Can you work these out from the drawing? Everything is in mm from the part's minimum corner. Coordinates: 2 decimals unless noted, no trailing zeros. Loops run counter-clockwise (first coordinate to the right, second up) from the corner with the lowest first, then second, coordinate; pieces in that order, holes last.
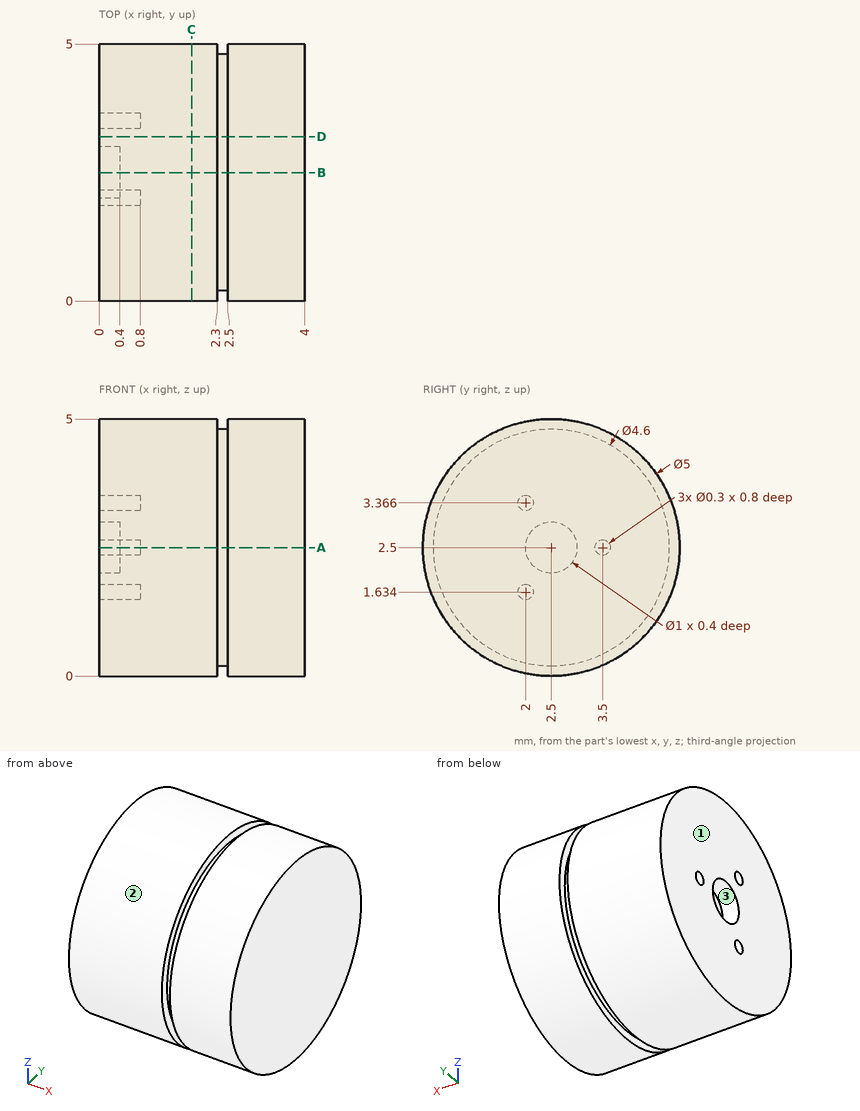
(1) We'd pull the mould along Z, two halves only. Please class the marked faces 1, 2 and 3: +Z half, -Z half, draft (parallel to the pull), parting line (faces both ways), or undercut.
Answers:
face 1: draft
face 2: parting line
face 3: undercut
(2) I need wall thicknesses on probe 1 along Y at (x, z) = (0.1, 2.5); probe 2 along Z at (x, y) = (0.3, 2.25); probe 3 along Z at (x, y) = (3.75, 2.6). Which ranges of each line are inside material? Lowest first, please.
Answers:
probe 1: y = 0 to 2, 3 to 3.35, 3.65 to 5
probe 2: z = 0.01 to 2.07, 2.93 to 4.99
probe 3: z = 0 to 5
(3) For pin 1 (0.5 mm diameter, centred on y = 2.5, z = 2.5, fed in from -X); pin 2 (2 mm diameter, centred on x = 3.5, z = 1, fed in from -Y), each with a flat end and sliding along its axis, tell me the tip position at first contact or that it passes through.
Answers:
pin 1: stops at x = 0.4
pin 2: stops at y = 0.05
(4) Imagine slicing it at A-A, the plane z = 2.5. Write out the boundary of the cut face in (x, y), and give its area (3 significant figures).
Answers:
outline: (0, 0) - (2.3, 0) - (2.3, 0.2) - (2.5, 0.2) - (2.5, 0) - (4, 0) - (4, 5) - (2.5, 5) - (2.5, 4.8) - (2.3, 4.8) - (2.3, 5) - (0, 5) - (0, 3.65) - (0.8, 3.65) - (0.8, 3.35) - (0, 3.35) - (0, 3) - (0.4, 3) - (0.4, 2) - (0, 2) - close
area: 19.3 mm2
(5) Imagine slicing it at C-C, the plane x = 1.8. Write out the boundary of the cut face in (y, z), and give its area (3 significant figures).
Answers:
outline: circle Ø5 at (2.5, 2.5)
area: 19.6 mm2
(6) Imagine slicing it at D-D, the plane y = 3.2. Write out the boundary of the cut face in (x, z), and give its area (3 significant figures).
Answers:
outline: (0, 0.1) - (2.3, 0.1) - (2.3, 0.31) - (2.5, 0.31) - (2.5, 0.1) - (4, 0.1) - (4, 4.9) - (2.5, 4.9) - (2.5, 4.69) - (2.3, 4.69) - (2.3, 4.9) - (0, 4.9) - close
area: 19.1 mm2
(7) Imagine slicing it at B-B, the plane y = 2.5. Write out the boundary of the cut face in (x, z), and give its area (3 significant figures).
Answers:
outline: (0, 0) - (2.3, 0) - (2.3, 0.2) - (2.5, 0.2) - (2.5, 0) - (4, 0) - (4, 5) - (2.5, 5) - (2.5, 4.8) - (2.3, 4.8) - (2.3, 5) - (0, 5) - (0, 3) - (0.4, 3) - (0.4, 2) - (0, 2) - close
area: 19.5 mm2
